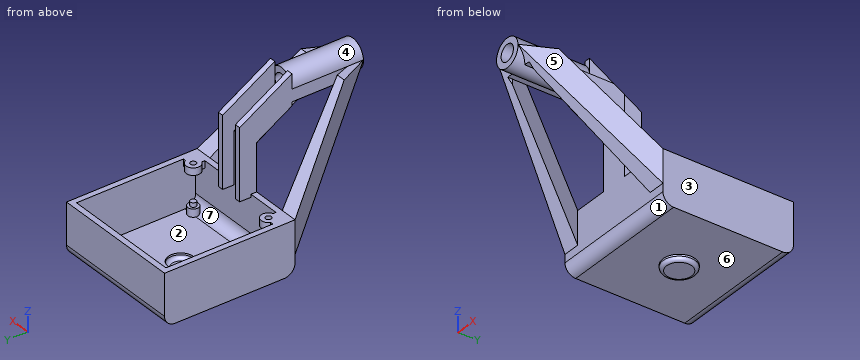
```python
from build123d import *
from build123d.topology import SkipClean

# Parameters (mm, degrees)
SKETCH1_W            = 36.5125
SKETCH1_H            = 36.5125
EXTRUDE1_DEPTH       = 1
SKETCH2_W            = 36.5125
SKETCH2_H            = 36.5125
SKETCH2_W_2          = 33.3375
SKETCH2_H_2          = 33.3375
EXTRUDE2_DEPTH       = 13.5
FILLET7_R            = 3
SKETCH5_R            = 1.5
EXTRUDE5_DEPTH       = 2.2
SKETCH6_R            = 0.8
EXTRUDE6_DEPTH       = 1.2
SKETCH7_R            = 4.5
EXTRUDE7_DEPTH       = 2.5
SKETCH8_R            = 3.5
EXTRUDE9_DEPTH       = 1.5
FILLET8_R            = 1
FILLET10_R           = 1
SKETCH9_R            = 0.4
EXTRUDE10_DEPTH      = 0.2
SKETCH10_R           = 0.8
EXTRUDE11_DEPTH      = 2
EXTRUDE12_DEPTH      = 19
EXTRUDE12_DEPTH_BACK = 0.8
EXTRUDE13_DEPTH      = 55.30808767
EXTRUDE14_DEPTH      = 17
EXTRUDE15_DEPTH      = 70.200859363
SKETCH16_R           = 4
SKETCH16_R_2         = 2.3
EXTRUDE16_DEPTH      = 20
SKETCH17_W           = 7.9375
SKETCH17_H           = 1.5875
EXTRUDE17_DEPTH      = 13.5
EXTRUDE18_START      = -1.5875
EXTRUDE18_DEPTH      = 15.875
EXTRUDE20_REACH      = 87.467
EXTRUDE21_DEPTH      = 1.5875
EXTRUDE22_REACH      = 88.701
EXTRUDE23_START      = -1.5875
EXTRUDE23_DEPTH      = 15.875
EXTRUDE24_REACH      = 87.467
EXTRUDE25_REACH      = 88.701
SKETCH25_W           = 14.2875
SKETCH25_H           = 28.3625
EXTRUDE26_DEPTH      = 1.5875
EXTRUDE27_DEPTH      = 1.613234818


with BuildPart() as part:
    # Sketch1 → Extrude1 (new body)
    with BuildSketch(Plane.XY):
        with Locations((18.25625, -18.25625)):
            Rectangle(SKETCH1_W, SKETCH1_H)
    extrude(amount=EXTRUDE1_DEPTH)

    # Sketch2 → Extrude2 (add)
    with BuildSketch(Plane.XY.offset(1)):
        with Locations((18.25625, -18.25625)):
            Rectangle(SKETCH2_W, SKETCH2_H)
        with Locations((18.25625, -18.25625)):
            Rectangle(SKETCH2_W_2, SKETCH2_H_2, mode=Mode.SUBTRACT)
    extrude(amount=EXTRUDE2_DEPTH)

    # Fillet7
    fillet7_edges = [part.edges().sort_by_distance(p)[0] for p in [
        (18.25625, -1.5875, 1),
        (18.25625, -34.925, 1),
        (18.25625, -36.5125, 0),
        (18.25625, 0, 0),
    ]]
    fillet(fillet7_edges, radius=FILLET7_R)

    # Sketch5 → Extrude5 (add)
    with BuildSketch(Plane.XY.offset(1)):
        with Locations(Location((4.25625, -4.25625, 0), (0, 0, 192.757983374))):
            Circle(SKETCH5_R)
        with Locations(Location((32.25625, -4.25625, 0), (0, 0, 192.757983374))):
            Circle(SKETCH5_R)
        with Locations(Location((4.25625, -32.25625, 0), (0, 0, 167.242016626))):
            Circle(SKETCH5_R)
        with Locations(Location((32.25625, -32.25625, 0), (0, 0, 167.242016626))):
            Circle(SKETCH5_R)
    extrude(amount=EXTRUDE5_DEPTH)

    # Sketch6 → Extrude6 (add)
    with BuildSketch(Plane.XY.offset(3.2)):
        with Locations((4.25625, -32.25625)):
            Circle(SKETCH6_R)
        with Locations((32.25625, -32.25625)):
            Circle(SKETCH6_R)
        with Locations((4.25625, -4.25625)):
            Circle(SKETCH6_R)
        with Locations((32.25625, -4.25625)):
            Circle(SKETCH6_R)
    extrude(amount=EXTRUDE6_DEPTH)

    # Sketch7 → Extrude7 (add)
    with BuildSketch(Plane.XY.offset(1)):
        with Locations((18.25625, -18.25625)):
            Circle(SKETCH7_R)
    extrude(amount=-EXTRUDE7_DEPTH)

    # Sketch8 → Extrude9 (cut)
    with BuildSketch(Plane.XY.offset(1)):
        with Locations((18.25625, -18.25625)):
            Circle(SKETCH8_R)
    extrude(amount=-EXTRUDE9_DEPTH, mode=Mode.SUBTRACT)

    # Fillet8
    fillet8_edges = [part.edges().sort_by_distance(p)[0] for p in [
        (13.75625, -18.25625, -1.5),
    ]]
    fillet(fillet8_edges, radius=FILLET8_R)

    # Fillet10
    fillet10_edges = [part.edges().sort_by_distance(p)[0] for p in [
        (14.75625, -18.25625, -0.5),
    ]]
    fillet(fillet10_edges, radius=FILLET10_R)

    # Sketch9 → Extrude10 (cut)
    with BuildSketch(Plane.XY.offset(-0.5)):
        with Locations((18.25625, -18.25625)):
            Circle(SKETCH9_R)
    extrude(amount=-EXTRUDE10_DEPTH, mode=Mode.SUBTRACT)

    # Sketch10 → Extrude11 (add)
    with BuildSketch(Plane.XY.offset(14.5)):
        with BuildLine():
            Line((31.5125, -34.11281563), (31.5125, -36.512569909))
            Line((31.5125, -36.512569909), (36.5125, -36.5125))
            Line((36.5125, -36.5125), (36.5125, -31.5125))
            Line((36.5125, -31.5125), (34.11281563, -31.5125))
            ThreePointArc((34.11281563, -31.5125), (30.842036438, -30.842036438), (31.5125, -34.11281563))
        make_face()
        with Locations((32.25625, -32.25625)):
            Circle(SKETCH10_R, mode=Mode.SUBTRACT)
        with BuildLine():
            Line((2.39968437, -31.5125), (0, -31.5125))
            Line((0, -31.5125), (0, -36.5125))
            Line((0, -36.5125), (5, -36.5125))
            Line((5, -36.5125), (5, -34.11281563))
            ThreePointArc((5, -34.11281563), (5.670463562, -30.842036438), (2.39968437, -31.5125))
        make_face()
        with Locations((4.25625, -32.25625)):
            Circle(SKETCH10_R, mode=Mode.SUBTRACT)
    extrude(amount=-EXTRUDE11_DEPTH)

    # Sketch11 → Extrude12 (add, two sides)
    with BuildSketch(Plane.XY.offset(14.5)) as extrude12_sk:
        Polygon((14.2875, -36.5125), (14.2875, -31.75), (15.875, -31.75), (15.875, -33.3375), (15.875, -34.925), (20.6375, -34.925), (20.6375, -33.3375), (20.6375, -31.75), (22.225, -31.75), (22.225, -36.5125), align=None)
    extrude(amount=EXTRUDE12_DEPTH)
    extrude(extrude12_sk.sketch, amount=-EXTRUDE12_DEPTH_BACK)

    # Sketch13 → Extrude13 (cut, through all)
    with BuildSketch(Plane.ZY.offset(-14.2875)):
        Polygon((33.5, -31.75), (25.5, -36.5125), (33.5, -36.5125), align=None)
    extrude(amount=-EXTRUDE13_DEPTH, mode=Mode.SUBTRACT)

    # Sketch14 → Extrude14 (add)
    with BuildSketch(Plane(origin=(0, -38.166778126, 22.721160103), x_dir=(1, 0, 0), z_dir=(0, -0.8592647834640841, 0.5115310664059621))):
        Polygon((22.225, 12.544258888), (22.225, 5.144258888), (14.2875, 5.144258888), (14.2875, 12.544258888), (15.875, 12.544258888), (15.875, 6.33740224), (20.6375, 6.33740224), (20.6375, 12.544258888), align=None)
    extrude(amount=EXTRUDE14_DEPTH)

    # Sketch15 → Extrude15 (cut, through all)
    with BuildSketch(Plane.ZY.offset(-14.2875)):
        Polygon((42.196028129, -46.357501319), (33.58401453, -46.357501319), (35.837468731, -50.14283121), align=None)
    extrude(amount=-EXTRUDE15_DEPTH, mode=Mode.SUBTRACT)

    # Sketch16 → Extrude16 (add)
    with BuildSketch(Plane.XZ.offset(46.357501319)):
        with Locations(Location((18.25625, 37.89002133, 0), (0, 0, 53.465087278))):
            Circle(SKETCH16_R)
        with Locations(Location((18.25625, 37.89002133, 0), (0, 0, 270))):
            Circle(SKETCH16_R_2, mode=Mode.SUBTRACT)
    extrude(amount=EXTRUDE16_DEPTH)

    # Sketch17 → Extrude17 (add)
    with BuildSketch(Plane.XY.offset(14.5)):
        with Locations((18.25625, -35.71875)):
            Rectangle(SKETCH17_W, SKETCH17_H)
    extrude(amount=EXTRUDE17_DEPTH)

    # Sketch18 → Extrude18 (add)
    with SkipClean():  # the faces are left unmerged after this step: merging them gives an invalid solid
        with BuildSketch(Plane.ZY.offset(-14.2875).offset(EXTRUDE18_START)):
            Polygon((38.1, -39.477034121), (38.1, -66.357501319), (3.495412711, -34.925), (35.390117188, -34.925), align=None)
        extrude(amount=EXTRUDE18_DEPTH)

    # Extrude20: up to this face of the body (flat: up to its plane)
    extrude20_end = Plane(part.part.faces().sort_by_distance((7.881670557, -51.329678598, 21.555608644))[0])
    # Sketch19 → Extrude20 (cut, up to the picked face)
    with BuildSketch(Plane.XY.offset(38.1), mode=Mode.PRIVATE) as extrude20_sk1:
        Polygon((0, -66.357501319), (14.261765182, -66.357501319), (0, -36.5125), align=None)
    extrude20_tool1 = split(extrude(extrude20_sk1.sketch, amount=-EXTRUDE20_REACH, mode=Mode.PRIVATE), bisect_by=extrude20_end, keep=Keep.BOTH, mode=Mode.PRIVATE)
    # Sketch19 → Extrude20 (cut, up to the picked face)
    with BuildSketch(Plane.XY.offset(38.1), mode=Mode.PRIVATE) as extrude20_sk2:
        Polygon((4.7625, -36.5125), (14.2875, -36.5125), (14.2875, -61.9125), align=None)
    extrude20_tool2 = split(extrude(extrude20_sk2.sketch, amount=-EXTRUDE20_REACH, mode=Mode.PRIVATE), bisect_by=extrude20_end, keep=Keep.BOTH, mode=Mode.PRIVATE)
    add(extrude20_tool1.solids().sort_by(Axis((4.753922, -56.409168, 38.1), (0, 0, -1)))[0], mode=Mode.SUBTRACT)
    add(extrude20_tool2.solids().sort_by(Axis((11.1125, -44.979167, 38.1), (0, 0, -1)))[0], mode=Mode.SUBTRACT)

    # Sketch20 → Extrude21 (cut)
    with SkipClean():  # the faces are left unmerged after this step: merging them gives an invalid solid
        with BuildSketch(Plane(origin=(15.875, 0, 0), x_dir=(0, 0, -1), z_dir=(1, 0, 0))):
            Polygon((-34.676044286, -63.247408093), (-33.89002133, -62.533437214), (-5.243119066, -36.5125), (-27.723162183, -36.5125), (-33.58401453, -46.357501319), (-33.89002133, -46.357501319), (-34.676044286, -46.357501319), align=None)
        extrude(amount=-EXTRUDE21_DEPTH, mode=Mode.SUBTRACT)

    # Extrude22: up to this plane
    with SkipClean():  # the faces are left unmerged after this step: merging them gives an invalid solid
        extrude22_end = Plane(origin=(4.7625, -36.5125, -19.465058372), z_dir=(-0.9363291775690445, -0.3511234415883917, 0))
        # Sketch21 → Extrude22 (cut, up to the surface)
        with BuildSketch(Plane.ZY, mode=Mode.PRIVATE) as extrude22_sk1:
            Polygon((38.1, -57.949167484), (38.1, -36.5125), (14.5, -36.5125), align=None)
        extrude22_tool1 = split(extrude(extrude22_sk1.sketch, amount=-EXTRUDE22_REACH, mode=Mode.PRIVATE), bisect_by=extrude22_end, keep=Keep.BOTH, mode=Mode.PRIVATE)
        add(extrude22_tool1.solids().sort_by_distance((0, -43.658056, 30.233333))[0], mode=Mode.SUBTRACT)

    # Sketch22 → Extrude23 (add)
    with BuildSketch(Plane(origin=(22.225, 0, 0), x_dir=(0, 0, -1), z_dir=(1, 0, 0)).offset(EXTRUDE23_START)):
        Polygon((-5.243119066, -36.5125), (-38.1, -66.357501319), (-38.1, -39.477034121), (-35.390117188, -34.925), (-4, -34.925), align=None)
    extrude(amount=EXTRUDE23_DEPTH)

    # Extrude24: up to this face of the body (flat: up to its plane)
    extrude24_end = Plane(part.part.faces().sort_by_distance((28.630829443, -51.329678598, 21.555608644))[0])
    # Sketch23 → Extrude24 (cut, up to the picked face)
    with BuildSketch(Plane.XY.offset(38.1), mode=Mode.PRIVATE) as extrude24_sk1:
        Polygon((22.250734818, -66.357501319), (36.5125, -66.357501319), (36.5125, -36.5125), align=None)
    extrude24_tool1 = split(extrude(extrude24_sk1.sketch, amount=-EXTRUDE24_REACH, mode=Mode.PRIVATE), bisect_by=extrude24_end, keep=Keep.BOTH, mode=Mode.PRIVATE)
    # Sketch23 → Extrude24 (cut, up to the picked face)
    with BuildSketch(Plane.XY.offset(38.1), mode=Mode.PRIVATE) as extrude24_sk2:
        Polygon((22.250734818, -61.84387382), (22.250734818, -36.5125), (31.75, -36.5125), align=None)
    extrude24_tool2 = split(extrude(extrude24_sk2.sketch, amount=-EXTRUDE24_REACH, mode=Mode.PRIVATE), bisect_by=extrude24_end, keep=Keep.BOTH, mode=Mode.PRIVATE)
    add(extrude24_tool1.solids().sort_by(Axis((31.758578, -56.409168, 38.1), (0, 0, -1)))[0], mode=Mode.SUBTRACT)
    add(extrude24_tool2.solids().sort_by(Axis((25.417157, -44.956291, 38.1), (0, 0, -1)))[0], mode=Mode.SUBTRACT)

    # Extrude25: up to this plane
    extrude25_end = Plane(origin=(31.75, -36.5125, -19.465058372), z_dir=(0.9363291775690447, -0.3511234415883913, 0))
    # Sketch24 → Extrude25 (cut, up to the surface)
    with BuildSketch(Plane(origin=(36.5125, 0, 0), x_dir=(0, 0, -1), z_dir=(1, 0, 0)), mode=Mode.PRIVATE) as extrude25_sk1:
        Polygon((-14.5, -36.5125), (-36.335175781, -36.5125), (-38.1, -39.477034121), (-38.1, -57.949167484), align=None)
    extrude25_tool1 = split(extrude(extrude25_sk1.sketch, amount=-EXTRUDE25_REACH, mode=Mode.PRIVATE), bisect_by=extrude25_end, keep=Keep.BOTH, mode=Mode.PRIVATE)
    add(extrude25_tool1.solids().sort_by_distance((36.5125, -43.722399, 30.157276))[0], mode=Mode.SUBTRACT)

    # Sketch25 → Extrude26 (cut)
    with BuildSketch(Plane(origin=(0, -34.925, 0), x_dir=(1, 0, 0), z_dir=(0, 1, 0))):
        with Locations((7.14375, -28.68125)):
            Rectangle(SKETCH25_W, SKETCH25_H)
        with Locations((29.36875, -28.68125)):
            Rectangle(SKETCH25_W, SKETCH25_H)
    extrude(amount=-EXTRUDE26_DEPTH, mode=Mode.SUBTRACT)

    # Sketch26 → Extrude27 (cut)
    with BuildSketch(Plane.ZY.offset(-20.6375)):
        Polygon((34.676044286, -46.357501319), (33.58401453, -46.357501319), (27.723162183, -36.5125), (5.243119066, -36.5125), (34.676044286, -63.247408093), align=None)
    extrude(amount=-EXTRUDE27_DEPTH, mode=Mode.SUBTRACT)


solid = part.part
```
The listing builds one solid part. Answer for the finished solid, in the listing's coordinates (mm). Face numbers are marked on the shaded views. A direction names the side the tool comes from. Round coordinates to 2 decimals unless told otherwise and drop trailing zeros. Write each loop counter-clockwise with the first axis right and the second up, starting at its lowest first coordinate (ties: lowest second). Pieces come first, ordered by that corner, then holes. Notation, with made-up numbers: (45.5, 47.25) -> (85.5, 47.25) arc R29 cw to (85.5, 67.25) -> close; hole circle Ø4 at (-4.5, 77.25). An arc over 180 degrees is marked (long way). Write item = value, one per line.
1) Straight lines are drawn through the part: line 1 along X through (y, z) = (-29.5, 8) (1 decimal); line 2 along Y through (x, z) = (15, 10) (1 decimal); line 3 along X through (y, z) = (-58.5, 34.5). For each, find the intervals that lie inside material, in ascending order. Write a range as [from, to].
Check values:
line_1 = [0, 1.6], [34.9, 36.5]
line_2 = [-36.5, -34.9], [-1.6, 0]
line_3 = [10.51, 13.01], [16.13, 20.38], [23.5, 26.01]
2) Section C-C on x = 11 is taken. Write down the section's boundary in (y, z) (1 decimal).
Check values:
outline = (-59.5, 30.6) -> (-53.1, 23.6) -> (-53.1, 32.8) -> (-57.9, 38.1) -> (-59.5, 38.1) -> close; (-36.5, 3) arc R3 ccw to (-33.5, 0) -> (-3, 0) arc R3 ccw to (0, 3) -> (0, 14.5) -> (-1.6, 14.5) -> (-1.6, 4) arc R3 cw to (-4.6, 1) -> (-31.9, 1) arc R3 cw to (-34.9, 4) -> (-34.9, 14.5) -> (-36.5, 14.5) -> close
3) Which of the six approach directions +Z, -Z, +X, -X, +Y, -Y give full straight-line access (tool end or side, diameter ignored) to the marked faces 4, 5, 6 and 7?
Check values:
face_4 = +Z, -Y
face_5 = +Z, -Z, +X, -Y
face_6 = -Z
face_7 = none
4) Given pin 1 (0.9 mm diameter, centred on x = 32.5, y = -4, fed in from +Z); pin 2 (2 mm diameter, centred on y = -36, z = 31.5, fed in from -X); pin 3 (1.4 mm diameter, centred on x = 19, z = 39.5, fed in from +Y), each flat-ended and moving along its own axis, determine where each tip first touches the part or whether it passes through.
Check values:
pin_1 = 4.4
pin_2 = 14.29
pin_3 = -46.36
5) Section D-D on y = -12.5 is taken. Write down the section's boundary in (x, z) (1 decimal).
Check values:
outline = (0, 0) -> (36.5, 0) -> (36.5, 14.5) -> (34.9, 14.5) -> (34.9, 1) -> (1.6, 1) -> (1.6, 14.5) -> (0, 14.5) -> close
6) Section A-A on y = -47.5 is taken. Give the number of separate pieces and of enclosed holes in the cut face, plus the area to 3 significant figures.
Check values:
separate_pieces = 3
enclosed_holes = 1
area = 104 mm²
7) For a pull along Y with two mould halves and no side action, classify the marked faces 1, 2 and 3 as released by +Y, released by -Y, zero draft, split by the parting line, or undercut.
Check values:
face_1 = released by -Y
face_2 = undercut
face_3 = zero draft
